Solid Edge part; units mm, degrees
sketch "Sketch1" plane through (0, 0, 0) normal (0, -1, 0) x (1, 0, 0)
  line L0 (-14, 36) -> (-42, 36)
  line L1 (-42, 36) -> (-42, -36)
  line L2 (-42, -36) -> (10, -36)
  arc A0 (10, -36) -> (42, -4) centre (10, -4) ccw
  line L3 (42, -4) -> (42, 13)
  arc A1 (27, 28) -> (42, 13) centre (27, 13) cw
  line L4 (10, 28) -> (27, 28)
  line L5 (10, -4) -> (10, 28)
  line L6 (-14, -4) -> (-14, 36)
  arc A2 (10, -4) -> (-14, -4) centre (-2, -4) cw
extrude "Protrusion1" add sketch "Sketch1" along normal mid plane 80
sketch "Sketch2" plane through (0, -40, 0) normal (0, -1, 0) x (1, 0, 0)
  line L0 (42, 0) -> (42, 28)
  line L1 (42, 28) -> (10, 28)
  line L2 (10, 28) -> (10, 0)
  line L3 (10, 0) -> (42, 0)
extrude "ExtrudedCutout_1" cut sketch "Sketch2" against normal blind 55
sketch "Sketch3" plane through (-28, 0, 36) normal (0, 0, 1) x (0, 1, 0)
  line L0 (0, -38) -> (40, -38)
  line L1 (40, -38) -> (40, 14)
  line L2 (40, 14) -> (0, 14)
  line L3 (0, 14) -> (0, -38)
extrude "ExtrudedCutout_2" cut sketch "Sketch3" against normal blind 72
sketch "Sketch4" plane through (-14, -20, 16) normal (1, 0, 0) x (0, 1, 0)
  line L0 (-12, 12) -> (-20, 12)
  line L1 (-20, 12) -> (-20, -4)
  line L2 (-20, -4) -> (-12, -4)
  line L3 (-12, -4) -> (-12, 12)
  line L4 (20, -5) -> (8, 20)
  line L5 (20, 20) -> (8, 20)
  line L6 (20, 20) -> (20, -5)
extrude "ExtrudedCutout_3" cut sketch "Sketch4" against normal blind 68.049
Design review of the part built by this model. Coordinates are the model's own, in mm. A direction names the side the tool comes from. Coordinates: 2 decimals unless noted, no trailing zeros. Write each loop counter-clockwise with the first axis right and the second up, starting at its lowest first coordinate (ties: lowest second). Pieces come first, ordered by that corner, then holes.
1) Insertion check: pin 1 (1 mm diameter, centred on x = 22.5, y = -29.5, fed in from -Z); pin 2 (3 mm diameter, centred on x = 20.5, z = 16.5, fed in from -Y); pin 3 (9.5 mm diameter, centred on x = 22.5, y = -23.5, fed in from +Z); pin 4 (12 mm diameter, centred on x = 11, y = 8, fed in from -Z). Each pin has a flat end and moves straight along its axis. Give the tip position at first contact, or say it passes through.
2) Mouldability with a two-part tool opening along Z and no side actions: class faces 1 (the flat face through (-28, -32, 20)), 2 (the cylindrical face through (-2, -20, -16)), 3 (the flat face through (-42, -20, 1)), 4 (the flat face through (-28, -36, 12)) as +Z half, -Z half, draft (parallel to the pull), parting line (faces both ways), or undercut.
3) Add section C-C (y = -25). Write out the cut boundary in (x, z).
4) Add section A-A (y = -34). Write out the cut boundary in (x, z), plus the area to 3 significant figures.
5) To check wall thickness, follow L1, parallel to Y at x = -32, z = -17; L2, parallel to X at y = -9, z = 15.5; L3, parallel to Y at x = 17, z = 2. State the ranges of each line that lie inside material, in increasing order.
6) Machinability: for faces 5 (the flat face through (26, -13, 0)), 6 (the flat face through (-14, -20, 16)), 7 (the flat face through (-28, -36, 28)), which of the approach directions +Z, -Z, +X, -X, +Y, -Y give a long, thin tool a straight path to every point of the face, cutting with its end or side? Answer none if there is none.
7) Add section B-B (z = 9.5). Write out the cut boundary in (x, y), plus the area to 3 significant figures.
8) Add section D-D (x = -31.5). Write out the cut boundary in (y, z).
Check result:
1. pin 1: stops at z = -33.66
1. pin 2: stops at y = 15
1. pin 3: stops at z = 0
1. pin 4: stops at z = -36
2. face 1: undercut
2. face 2: +Z half
2. face 3: draft
2. face 4: undercut
3. outline: (-42, -36) - (10, -36) arc R32 ccw to (42, -4) - (42, 0) - (10, 0) - (10, -4) arc R12 cw to (-14, -4) - (-14, 36) - (-42, 36) - close
4. outline: (-42, -36) - (10, -36) arc R32 ccw to (42, -4) - (42, 0) - (10, 0) - (10, -4) arc R12 cw to (-14, -4) - (-14, 12) - (-42, 12) - close; (-42, 28) - (-14, 28) - (-14, 36) - (-42, 36) - close
4. area: 3,040 mm2
5. L1: y = -40 to 0
5. L2: x = -42 to -14
5. L3: y = 15 to 40
6. face 5: +Z, +X, -Y
6. face 6: +Z, +Y, -Y
6. face 7: +X, -X, -Y
7. outline: (-42, -40) - (-14, -40) - (-14, 0) - (-42, 0) - close; (10, 15) - (42, 15) - (42, 40) - (10, 40) - close
7. area: 1,920 mm2
8. outline: (-40, -36) - (0, -36) - (0, 11) - (-12, 36) - (-40, 36) - (-40, 28) - (-32, 28) - (-32, 12) - (-40, 12) - close
